Geometry: see drawing. Coordinates: mm, zero at the bounding-box minimum. A direction names the side the tool comes from. Round coordinates to 2 decimals unless told otherwise and drop trailing zeros. Write each loop counter-clockwise with the first axis right and the second up, starting at its lowest first coordinate (ties: lowest second). Pieces come first, ordered by that corner, then holes. Notation, with made-up numbers: M -12.5,53 L -8.5,53 A32 ccw -8.5,90 Z; hole C 32,71.25 d11. An arc over 180 degrees is marked long. Use a Markdown table: item, result.
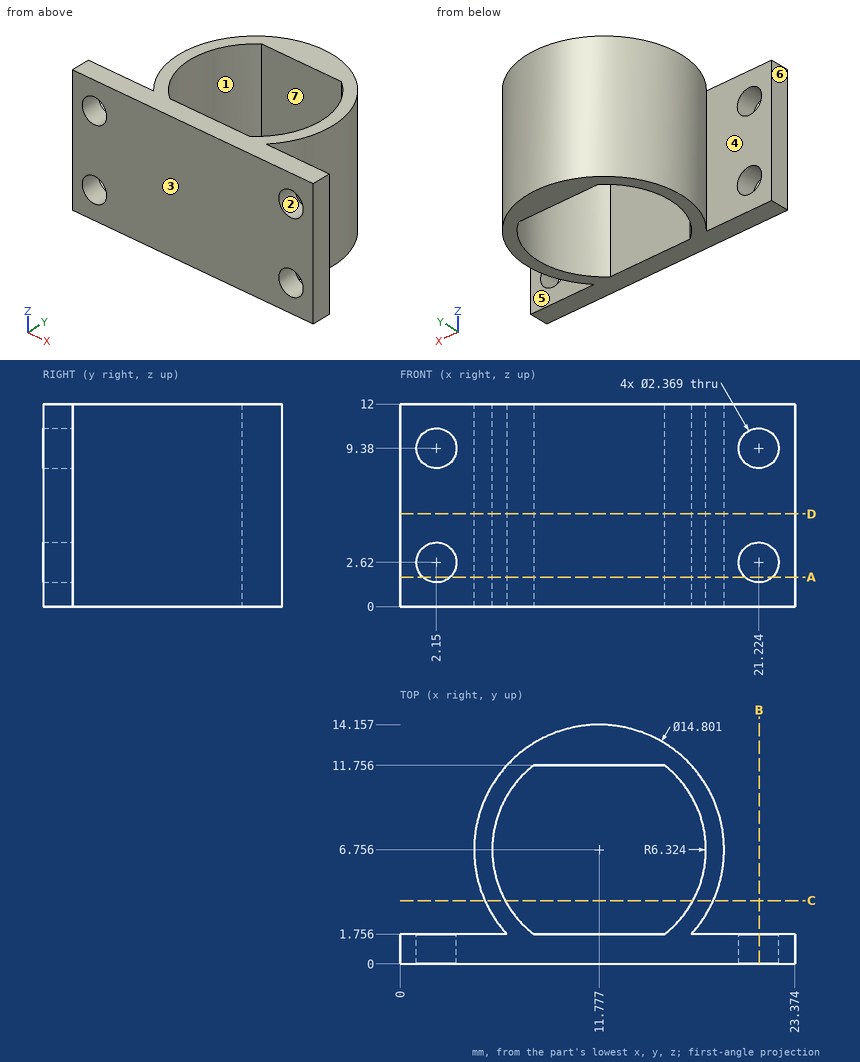
Q1. Section C-C on y = 3.75. Return loops of the section in (x, z) (1 decimal).
Results are:
| item | result |
|---|---|
| outline | M 5,0 L 6.2,0 L 6.2,12 L 5,12 Z; M 17.3,0 L 18.5,0 L 18.5,12 L 17.3,12 Z |
Q2. Line query: L1, parallel to X at y = 11.5, z = 11.5 (1 decimal); L2, parallel to X at y = 6.5, z = 7.5 (1 decimal); L3, parallel to Y at x = 12, z = 4.25. Output: solid intervals per line, ascending.
Results are:
| item | result |
|---|---|
| L1 | 6.1 to 7.6, 16 to 17.5 |
| L2 | 4.4 to 5.5, 18.1 to 19.2 |
| L3 | 0 to 1.76, 11.76 to 14.15 |
Q3. Reachability of the marked faces 4, 5, 6 and 7 from +Z, -Z, +X, -X, +Y, -Y: full face, straight path, thin tool, end or side. Return the list, or none.
Results are:
| item | result |
|---|---|
| face 4 | +Z, -Z, -X |
| face 5 | +Z, -Z, +X |
| face 6 | +Z, -Z, -X, +Y, -Y |
| face 7 | +Z, -Z |
Q4. Section D-D on z = 5.5. Return loops of the section in (x, y) (1 decimal).
Results are:
| item | result |
|---|---|
| outline | M 0,0 L 23.4,0 L 23.4,1.8 L 17.2,1.8 A7.4 ccw long 6.3,1.8 L 0,1.8 Z; hole M 7.9,1.8 L 15.6,1.8 A6.3 ccw 15.6,11.8 L 7.9,11.8 A6.3 ccw Z |
Q5. Mould query, pull axis Y, two halves, no side actions, for the marked faces 1, 2 and 3. Classes: +Y half, -Y half, draft (parallel to the pull), parting line (faces both ways), or undercut.
Results are:
| item | result |
|---|---|
| face 1 | undercut |
| face 2 | draft |
| face 3 | -Y half |
Q6. Section B-B on x = 21.25. Return loops of the section in (y, z) (1 decimal).
Results are:
| item | result |
|---|---|
| outline | M 0,0 L 1.8,0 L 1.8,1.4 L 0,1.4 Z; M 0,3.8 L 1.8,3.8 L 1.8,8.2 L 0,8.2 Z; M 0,10.6 L 1.8,10.6 L 1.8,12 L 0,12 Z |
Q7. First-contact query: pin 1 Ø1.5 at (y, z) = (3.5, 11) entering from -X; pin 2 Ø5 at (x, z) = (4.5, 8.5) entering from +Y; pin 3 Ø1.9 at (x, z) = (2.15, 9.38) entering from -Y; pin 4 Ø7 at (x, z) = (20, 4) entering from +Y (1 decimal). Flat tips, straight axial feed; report the tip coordinate or a pass-through.
Results are:
| item | result |
|---|---|
| pin 1 | x = 4.81 |
| pin 2 | y = 12.41 |
| pin 3 | through |
| pin 4 | y = 12.5 |
Q8. Section A-A on z = 1.75. Return loops of the section in (x, y) (1 decimal).
Results are:
| item | result |
|---|---|
| outline | M 0,0 L 1.3,0 L 1.3,1.8 L 0,1.8 Z; M 3,0 L 20.4,0 L 20.4,1.8 L 17.2,1.8 A7.4 ccw long 6.3,1.8 L 3,1.8 Z; M 22,0 L 23.4,0 L 23.4,1.8 L 22,1.8 Z; hole M 7.9,1.8 L 15.6,1.8 A6.3 ccw 15.6,11.8 L 7.9,11.8 A6.3 ccw Z |
